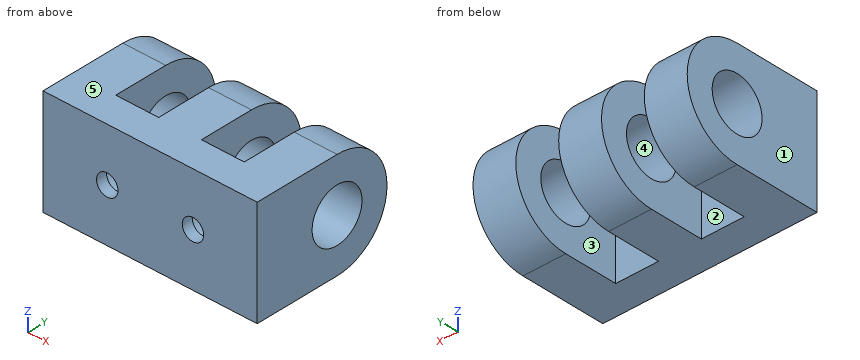
Autodesk Fusion 360 part; units mm, degrees
sketch "Sketch1" plane through (0, 0, 0) normal (0, 1, 0) x (1, 0, 0)
  line L0 (50, -25) -> (-50, -25)
  line L1 (-50, -25) -> (-50, 25)
  line L2 (-50, 25) -> (50, 25)
  line L3 (50, 25) -> (50, -25)
  line L4 (50, -25) -> (-50, 25) construction
  line L5 (-50, -25) -> (50, 25) construction
  dimension "d1" = 100
  dimension "d2" = 50
extrude "Extrude1" add sketch "Sketch1" along normal blind 65
sketch "Sketch2" plane through (0, 0, 25) normal (0, 0, 1) x (1, 0, 0)
  line L0 (-50, 0) -> (50, 0)
  line L1 (50, 0) -> (50, 65)
  line L2 (50, 65) -> (-50, 65)
  line L3 (-50, 65) -> (-50, 0)
  line L4 (-50, 0) -> (50, 0)
  line L5 (50, 0) -> (50, 15)
  line L6 (50, 15) -> (-50, 15)
  line L7 (-50, 15) -> (-50, 0)
  line L8 (-40, 15) -> (-50, 15)
  line L9 (-50, 15) -> (-50, 65)
  line L10 (-50, 65) -> (-40, 65)
  line L11 (40, 15) -> (50, 15)
  line L12 (50, 15) -> (50, 65)
  line L13 (50, 65) -> (40, 65)
  line L14 (-10, 65) -> (10, 65)
  line L15 (10, 65) -> (10, 15)
  line L16 (10, 15) -> (-10, 15)
  line L17 (-10, 15) -> (-10, 65)
  line L18 (10, 65) -> (30, 65)
  line L19 (30, 65) -> (30, 15)
  line L20 (30, 15) -> (10, 15)
  line L21 (10, 15) -> (10, 65)
  line L22 (-10, 65) -> (-30, 65)
  line L23 (-30, 65) -> (-30, 15)
  line L24 (-30, 15) -> (-10, 15)
  line L25 (-10, 15) -> (-10, 65)
  line L26 (-30, 65) -> (-50, 65)
  line L27 (-50, 65) -> (-50, 15)
  line L28 (-50, 15) -> (-30, 15)
  line L29 (-30, 15) -> (-30, 65)
  line L30 (30, 65) -> (50, 65)
  line L31 (50, 65) -> (50, 15)
  line L32 (50, 15) -> (30, 15)
  line L33 (30, 15) -> (30, 65)
  dimension "d5" = 100
  dimension "d6" = 15
  dimension "d7" = 20
  dimension "d8" = 20
  dimension "d9" = 20
  dimension "d10" = 20
  dimension "d11" = 20
extrude "Extrude2" cut sketch "Sketch2" against normal blind 50 contours L2 L6 L17 L22 L23 L24 L25 L29 | L2 L6 L15 L18 L19 L20 L21 L33
sketch "Sketch3" plane through (-50, 0, 0) normal (-1, 0, 0) x (0, 0, 1)
  line L0 (-25, 0) -> (25, 0)
  line L1 (25, 0) -> (25, 65)
  line L2 (25, 65) -> (-25, 65)
  line L3 (-25, 65) -> (-25, 0)
  circle A0 centre (0, 40) radius 25
  dimension "d14" = 50
  dimension "d15" = 40
extrude "Extrude3" cut sketch "Sketch3" against normal blind 100 contours L2 L3 A0 | L1 L2 A0
sketch "Sketch4" plane through (-50, 0, 0) normal (-1, 0, 0) x (0, 0, 1)
  arc A0 (25, 40) -> (-25, 40) centre (0, 40) ccw
  line L0 (-25, 40) -> (-25, 0)
  line L1 (-25, 0) -> (25, 0)
  line L2 (25, 0) -> (25, 40)
  line L3 (0, 40) -> (0, 0)
hole "Hole1" at (-50, 40, 0) direction (1, 0, 0) diameter 25 end through all
sketch "Sketch5" plane through (0, 15, 0) normal (0, 1, 0) x (-1, 0, 0)
  line L0 (30, 25) -> (10, 25)
  line L1 (10, 25) -> (10, -25)
  line L2 (10, -25) -> (30, -25)
  line L3 (30, -25) -> (30, 25)
  line L4 (20, 0) -> (20, -25)
  line L5 (-20, 0) -> (-20, -25)
  dimension "d21" = 25
  dimension "d22" = 40
hole "Hole2" at (-20, 15, 0) at (20, 15, 0) direction (0, -1, 0) diameter 10 depth 100 tip angle 118 counterbore diameter 16 counterbore depth 10
The model under review builds one solid part; all positions refer to its coordinate system, in mm. Face numbers are marked on the shaded views. A direction names the side the tool comes from. Round coordinates to 2 decimals unless told otherwise and drop trailing zeros. Order: outer loops, then holes, each group sorted by start corner. A loop starts at its lowest first (then second) coordinate and runs counter-clockwise, first axis right, second up.
Item 1: For pin 1 (25 mm diameter, centred on y = 33, z = -8, fed in from -X); pin 2 (6 mm diameter, centred on x = -22.5, z = -8, fed in from +Y); pin 3 (16 mm diameter, centred on x = 24, z = 8, fed in from +Y), all flat-tipped, find the tip position at first contact; note any pin that passes through.
Working result:
pin 1: stops at x = -50
pin 2: stops at y = 15
pin 3: stops at y = 64.85
Item 2: Draft analysis for pull direction Z (two halves, no side actions). For the marked faces 3, 4 and 5, state which applies: released by +Z, released by -Z, zero draft, split by the parting line, or undercut.
Working result:
face 3: zero draft
face 4: undercut
face 5: released by +Z
Item 3: Machinability: for the marked faces 1 and 2, which of the approach directions +Z, -Z, +X, -X, +Y, -Y give a long, thin tool a straight path to every point of the face, cutting with its end or side? Answer none if there is none.
Working result:
face 1: +Z, -Z, -X, +Y, -Y
face 2: +Z, -Z, +Y
Item 4: To check wall thickness, follow probe 1 along X at (y, z) = (19, -14.5); probe 2 along X at (y, z) = (1.7, 0); probe 3 along Y at (x, z) = (39, 0). State the ranges of each line that lie inside material, in increasing order.
Working result:
probe 1: x = -50 to -30, -10 to 10, 30 to 50
probe 2: x = -50 to -25, -15 to 15, 25 to 50
probe 3: y = 0 to 27.5, 52.5 to 65
Item 5: Add section C-C, the plane x = 8. State the section outline as (y, z) points, and give its area (3 significant figures).
Working result:
outline: (0, -25) - (40, -25) arc R25 ccw to (40, 25) - (0, 25) - close; hole circle Ø25 at (40, 0)
area: 2,490 mm2
Item 6: Add section A-A, the plane x = -20. State the section outline as (y, z) points.
Working result:
outline: (0, -25) - (15, -25) - (15, -8) - (5, -8) - (5, -5) - (0, -5) - close; (0, 5) - (5, 5) - (5, 8) - (15, 8) - (15, 25) - (0, 25) - close
Item 7: Add section D-D, the plane y = 6.5. State the section outline as (x, z) points.
Working result:
outline: (-50, -25) - (50, -25) - (50, 25) - (-50, 25) - close; hole circle Ø16 at (-20, 0); hole circle Ø16 at (20, 0)
Item 8: Add section B-B, the plane y = 55.5. State the section outline as (x, z) points.
Working result:
outline: (-50, -19.62) - (-30, -19.62) - (-30, 19.62) - (-50, 19.62) - close; (-10, -19.62) - (10, -19.62) - (10, 19.62) - (-10, 19.62) - close; (30, -19.62) - (50, -19.62) - (50, 19.62) - (30, 19.62) - close
